Geometry: final body of the model. Coordinates: model frame, mm. A direction names the side the tool comes from. Round coordinates to 2 decimals unless told otherwise and drop trailing zeros. Loops run counter-clockwise (first coordinate to the right, second up) from the corner with the lowest first, then second, coordinate; pieces in that order, holes last. Notation, with made-up numbers: (-36.5, 21) - (0.5, 21) arc R16 ccw to (0.5, 41) - close; hole circle Ø1 at (-2, 76.25). An arc over 180 degrees is marked (long way). Answer as CSV lines item,"result".
Autodesk Inventor part; units mm, degrees
ref_plane "tnut_XY" through (0, 0, -1.1938) normal (0, 0, 1) x (1, 0, 0)
ref_plane "tnut_YZ" through (0, 0, -1.1938) normal (1, 0, 0) x (0, 1, 0)
ref_plane "tnut_ZX" through (0, 0, -1.1938) normal (0, 1, 0) x (0, 0, 1)
sketch "Sketch_1" plane through (0, 0, 0) normal (0, 0, 1) x (1, 0, 0)
  arc A0 (-5.4864, 5.6261) -> (-5.4864, -5.6261) centre (-5.4864, 0) ccw
  line L0 (-5.4864, -5.6261) -> (5.4864, -5.6261)
  arc A1 (5.4864, -5.6261) -> (5.4864, 5.6261) centre (5.4864, 0) ccw
  line L1 (5.4864, 5.6261) -> (-5.4864, 5.6261)
extrude "Extrusion1" add sketch "Sketch_1" along normal mid plane 2.3876
sketch "Sketch_3" plane through (0, 0, 0) normal (0, 0, 1) x (1, 0, 0)
  circle A0 centre (0, 0) radius 2.5781
extrude "Extrusion2" add sketch "Sketch_3" along normal blind 1.9558
sketch "Sketch_4" plane through (0, 0, 0) normal (1, 0, 0) x (0, 1, 0)
  line L0 (0, -1.1938) -> (0, 1.9558)
  line L1 (0, 1.9558) -> (2.0828, 1.9558)
  line L2 (2.0828, 1.9558) -> (1.6535, 1.5265)
  line L3 (1.6535, 1.5265) -> (1.6535, -0.7645)
  line L4 (1.6535, -0.7645) -> (2.0828, -1.1938)
  line L5 (2.0828, -1.1938) -> (0, -1.1938)
  line L6 (0, -1.1938) -> (0, 1.9558)
revolve "Revolution1" cut sketch "Sketch_4" angle 360 about axis through (0, 0, -1.1938) along (0, 0, -1)
thread "Thread1"
ref_plane "tnut_XY" through (0, 0, -1.1938) normal (0, 0, 1) x (1, 0, 0)
ref_plane "tnut_YZ" through (0, 0, -1.1938) normal (1, 0, 0) x (0, 1, 0)
ref_plane "tnut_ZX" through (0, 0, -1.1938) normal (0, 1, 0) x (0, 0, 1)
ref_plane "tnut1_XY" through (0, 0, 1.1938) normal (0, 0, 1) x (1, 0, 0)
ref_plane "tnut1_YZ" through (0, 0, 1.1938) normal (1, 0, 0) x (0, 1, 0)
ref_plane "tnut1_ZX" through (0, 0, 1.1938) normal (0, 1, 0) x (0, 0, 1)
properties part number "3275"
(1) Section A-A (x = 0). Output: boundary loops of the cut face in (y, z).
Findings below:
outline,"(-5.63, -1.19) - (-2.08, -1.19) - (-1.65, -0.76) - (-1.65, 1.53) - (-2.08, 1.96) - (-2.58, 1.96) - (-2.58, 1.19) - (-5.63, 1.19) - close; (1.65, -0.76) - (2.08, -1.19) - (5.63, -1.19) - (5.63, 1.19) - (2.58, 1.19) - (2.58, 1.96) - (2.08, 1.96) - (1.65, 1.53) - close"
(2) Section C-C (x = -3.5). Output: boundary loops of the cut face in (y, z).
Findings below:
outline,"(-5.63, -1.19) - (5.63, -1.19) - (5.63, 1.19) - (-5.63, 1.19) - close"
(3) Section D-D (y = 4). Output: boundary loops of the cut face in (x, z), and give its area (3 significant figures).
Findings below:
outline,"(-9.44, -1.19) - (9.44, -1.19) - (9.44, 1.19) - (-9.44, 1.19) - close"
area,"45.1 mm2"
(4) Draft query along Y for faces 3 (the face through (0, 3, 1.194)), 4 (the face through (11.11, 0.12, -0.02)), 5 (the face through (-1.01, -1.31, 0.36)), 6 (the face through (0, -5.626, 0)). Return one class per face: pulls with the +Y half, pulls with the -Y half, needs draft (parallel to the pull), parting line crosses it, or undercut.
Findings below:
face 3,"needs draft"
face 4,"parting line crosses it"
face 5,"undercut"
face 6,"pulls with the -Y half"
(5) Access query for faces 1 (the face through (1.39, -2.17, 1.57)), 2 (the face through (2.3, 0.1, -1.194)). Directions: +Z, -Z, +X, -X, +Y, -Y. A direction counts if a zero-diameter tool reaches every point of the face in a straight line with its end or side. Return the directions, or none.
Findings below:
face 1,"+Z"
face 2,"-Z, +X, -X, +Y, -Y"
(6) Material intervals for line 1 along X through (y, z) = (0, 1); line 2 along Z through (x, y) = (2, -4); line 3 along Y through (x, z) = (1, -0.7), sorted ascending.
Findings below:
line 1,"-11.11 to -1.65, 1.65 to 11.11"
line 2,"-1.19 to 1.19"
line 3,"-5.63 to -1.32, 1.32 to 5.63"
(7) Section B-B (y = 0). Output: boundary loops of the cut face in (x, z), and give its area (3 significant figures).
Findings below:
outline,"(-11.11, -1.19) - (-2.08, -1.19) - (-1.65, -0.76) - (-1.65, 1.53) - (-2.08, 1.96) - (-2.58, 1.96) - (-2.58, 1.19) - (-11.11, 1.19) - close; (1.65, -0.76) - (2.08, -1.19) - (11.11, -1.19) - (11.11, 1.19) - (2.58, 1.19) - (2.58, 1.96) - (2.08, 1.96) - (1.65, 1.53) - close"
area,"46.2 mm2"
(8) Pin query (flat end, axial travel): P1, Ø1.5, axis at y = -2, z = 0.5, coming from the +X side. Return the tip coordinate at first contact, or that it passes through.
Findings below:
P1,"x = 10.97"
